For this review, take the finished solid that the model builds, in its own axes (mm). Face numbers are marked on the shaded views. Coordinates: 2 decimals unless noted, no trailing zeros. Loops run counter-clockwise (first coordinate to the right, second up) from the corner with the lowest first, then second, coordinate; pieces in that order, holes last. Notation, with made-up numbers: (-39.5, 11) -> (-0.5, 11) arc R14 ccw to (-0.5, 24) -> close; hole circle Ø10 at (59.25, -4.75). An arc over 180 degrees is marked (long way). Use a Markdown table: item, result.
from build123d import *

# Parameters (mm, degrees)
F1_DEPTH = 9
F3_R     = 1.4
F4_DEPTH = 25
F2_R     = 2.5
F5_DEPTH = 25


with BuildPart() as f1:
    # F0 (on Top) → F1 (new body)
    with BuildSketch(Plane.XY):
        Polygon((-5, -4.5), (10, -4.5), (10, 0), (10, 4.5), (-15, 4.5), (-15, -2.5), (-15, -4.5), align=None)
    extrude(amount=F1_DEPTH)

    # F3 (on face) → F4 (cut)
    with BuildSketch(Plane.XY.offset(9)):
        with Locations((-12, 0)):
            Circle(F3_R)
    extrude(amount=-F4_DEPTH, mode=Mode.SUBTRACT)

    # F2 (on face) → F5 (cut)
    with BuildSketch(Plane.YZ.offset(10)):
        with Locations((0, 4.5)):
            Circle(F2_R)
    extrude(amount=-F5_DEPTH, mode=Mode.SUBTRACT)


solid = f1.part
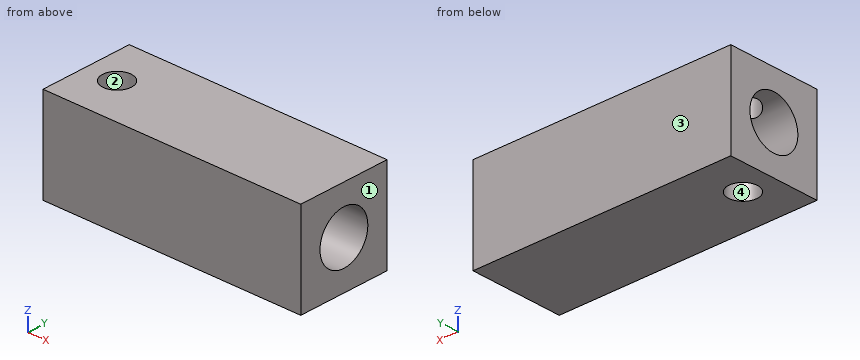
(1) For line 1 along X through (y, z) = (0, 7.15); line 2 along Z through (x, y) = (-0.75, 0); line 3 along Y through (x, z) = (-12, 7.65), list the stretches that pass through material, from the lowest coordinate up.
Found:
| item | result |
|---|---|
| line 1 | x = -15 to -13.4, -10.6 to 10 |
| line 2 | z = 0 to 2, 7 to 9 |
| line 3 | y = -4.5 to -1.4, 1.4 to 4.5 |
(2) Take a section at C-C on y = 0. Write out the cut boundary in (x, z), plus the area to 3 significant figures.
Found:
| item | result |
|---|---|
| outline | (-15, 0) -> (-13.4, 0) -> (-13.4, 2) -> (-15, 2) -> close; (-15, 7) -> (-13.4, 7) -> (-13.4, 9) -> (-15, 9) -> close; (-10.6, 0) -> (10, 0) -> (10, 2) -> (-10.6, 2) -> close; (-10.6, 7) -> (10, 7) -> (10, 9) -> (-10.6, 9) -> close |
| area | 88.8 mm^2 |
(3) Take a section at A-A on x = -12. Write out the cut boundary in (y, z), plus the area to 3 significant figures.
Found:
| item | result |
|---|---|
| outline | (-4.5, 0) -> (-1.4, 0) -> (-1.4, 2.43) arc R2.5 cw to (-1.4, 6.57) -> (-1.4, 9) -> (-4.5, 9) -> close; (1.4, 0) -> (4.5, 0) -> (4.5, 9) -> (1.4, 9) -> (1.4, 6.57) arc R2.5 cw to (1.4, 2.43) -> close |
| area | 49.4 mm^2 |
(4) Mouldability with a two-part tool opening along X and no side actions: class the marked faces 1, 2, 3 and 4 as pulls with the +X half, pulls with the -X half, needs draft (parallel to the pull), parting line crosses it, or undercut.
Found:
| item | result |
|---|---|
| face 1 | pulls with the +X half |
| face 2 | undercut |
| face 3 | needs draft |
| face 4 | undercut |
(5) Take a section at B-B on z = 4.5. Write out the cut boundary in (x, y).
Found:
| item | result |
|---|---|
| outline | (-15, -4.5) -> (10, -4.5) -> (10, -2.5) -> (-15, -2.5) -> close; (-15, 2.5) -> (10, 2.5) -> (10, 4.5) -> (-15, 4.5) -> close |
(6) Take a section at D-D on y = -1.75. Write out the cut boundary in (x, z).
Found:
| item | result |
|---|---|
| outline | (-15, 0) -> (10, 0) -> (10, 2.71) -> (-15, 2.71) -> close; (-15, 6.29) -> (10, 6.29) -> (10, 9) -> (-15, 9) -> close |
